For this review, take the finished solid that the model builds, in its own axes (mm). A direction names the side the tool comes from. Give positions to 0.01 mm unless a question says otherwise; leave off trailing zeros. Loops run counter-clockwise (first coordinate to the right, second up) from the corner with the lowest first, then second, coordinate; pieces in that order, holes last. Notation, with made-up numbers: (1, 26) -> (29, 26) arc R19 ccw to (29, 31) -> close; hole circle Ø3 at (-0.75, 37). An arc over 180 degrees is marked (long way). One line per question, with ' | ' between items. Start each with the question number.
(1) Consider section A-A (y = 6.5). Write out the cut boundary in (x, z), and give its area (3 significant figures).
(2) Wall thickness on probe 1 along Z at (x, y) = (-5.5, 11.25); probe 2 along Z at (x, y) = (0.25, 10.5); probe 3 along X at (y, z) = (12.3, 6.25): over which ranges is each line inside the solid? List them lowest first.
(3) Tool access review of faces 1 (the flat face through (-1, 3, -6)), 2 (the cylindrical face through (0.13, 12.73, 5.26)), 3 (the cylindrical face through (-3.361, 4.473, 11.186)): name each direction out of +Z, -Z, +X, -X, +Y, -Y from which nothing blocks a thin tool from reaching the whole face with its end or side.
(4) Insertion check: P1, Ø1, axis at x = -5.5, y = 9.5, coming from the -Z side; P2, Ø3, axis at x = -3.5, y = 11, coming from the +Z side; P3, Ø0.6, axis at y = 13, z = 0.5, coming from the -X side. Each pin has a flat end and moves straight along its axis. Give the tip position at first contact, or say it passes through.
from build123d import *

# Parameters (mm, degrees)
SKETCH1_W                    = 8.5
SKETCH1_H                    = 14.5
CUT_EXTRUDE1_REACH           = 2.1
CUT_EXTRUDE2_REACH           = 2.1
CUT_EXTRUDE3_REACH           = 2.1
CUT_EXTRUDE4_REACH           = 2.1
F_2_0_2_DIAMETER_HOLE1_D     = 2
F_2_0_2_DIAMETER_HOLE1_DEPTH = 3
F_2_0_2_DIAMETER_HOLE2_D     = 2
F_2_0_2_DIAMETER_HOLE2_DEPTH = 3.5
F_2_0_2_DIAMETER_HOLE3_D     = 2
F_2_0_2_DIAMETER_HOLE3_DEPTH = 3
F_2_0_2_DIAMETER_HOLE4_D     = 2
F_2_0_2_DIAMETER_HOLE4_DEPTH = 3.5


with BuildPart() as part:
    # Sketch1 → Revolve1 (revolve)
    with BuildSketch(Plane(origin=(0, 0, 0), x_dir=(-1, 0, 0), z_dir=(0, 0, -1))):
        with Locations((-4.25, 7.25)):
            Rectangle(SKETCH1_W, SKETCH1_H)
    revolve(axis=Axis((0, 0, 0), (0, 1, 0)))

    # Sketch2 → Cut-Extrude1 (cut, up to next)
    with BuildSketch(Plane(origin=(-8.4, 0, 0), x_dir=(0, 0, -1), z_dir=(1, 0, 0)), mode=Mode.PRIVATE) as cut_extrude1_sk1:
        Polygon((0.9, 13.234042555), (0.9, 13.297872335), (0.649999993, 13.297872335), (0.649999993, 13.553191453), (0.587500007, 13.553191453), (0.587500007, 13.297872335), (0.3375, 13.297872335), (0.3375, 13.234042555), (0.587500007, 13.234042555), (0.587500007, 12.978723392), (0.649999993, 12.978723392), (0.649999993, 13.234042555), align=None)
    cut_extrude1_tool1 = extrude(cut_extrude1_sk1.sketch, amount=-CUT_EXTRUDE1_REACH, mode=Mode.PRIVATE) & part.part
    add(cut_extrude1_tool1.solids().sort_by_distance((-8.4, 13.265957, -0.61875))[0], mode=Mode.SUBTRACT)

    # Sketch3 → Cut-Extrude2 (cut, up to next)
    with BuildSketch(Plane.XY.offset(-8.4), mode=Mode.PRIVATE) as cut_extrude2_sk1:
        Polygon((1, 13.234042555), (1, 13.297872335), (0.749999993, 13.297872335), (0.749999993, 13.553191453), (0.687500007, 13.553191453), (0.687500007, 13.297872335), (0.4375, 13.297872335), (0.4375, 13.234042555), (0.687500007, 13.234042555), (0.687500007, 12.978723392), (0.749999993, 12.978723392), (0.749999993, 13.234042555), align=None)
    cut_extrude2_tool1 = extrude(cut_extrude2_sk1.sketch, amount=-CUT_EXTRUDE2_REACH, mode=Mode.PRIVATE) & part.part
    add(cut_extrude2_tool1.solids().sort_by_distance((0.71875, 13.265957, -8.4))[0], mode=Mode.SUBTRACT)

    # Sketch4 → Cut-Extrude3 (cut, up to next)
    with BuildSketch(Plane.XY.offset(-8.4), mode=Mode.PRIVATE) as cut_extrude3_sk1:
        Polygon((-0.875, 12.5), (-0.43749997, 13.106382996), (-3e-08, 12.5), (0.18749997, 12.5), (-0.34374997, 13.265957445), (0.18749997, 14), (-3e-08, 14), (-0.43749997, 13.393617004), (-0.875, 14), (-1.0625, 14), (-0.53125006, 13.265957445), (-1.0625, 12.5), align=None)
    cut_extrude3_tool1 = extrude(cut_extrude3_sk1.sketch, amount=-CUT_EXTRUDE3_REACH, mode=Mode.PRIVATE) & part.part
    add(cut_extrude3_tool1.solids().sort_by_distance((-0.4375, 13.242259, -8.4))[0], mode=Mode.SUBTRACT)

    # Sketch5 → Cut-Extrude4 (cut, up to next)
    with BuildSketch(Plane(origin=(-8.4, 0, 0), x_dir=(0, 0, -1), z_dir=(1, 0, 0)), mode=Mode.PRIVATE) as cut_extrude4_sk1:
        Polygon((-1.10000006, 14), (-0.6, 13.265957445), (-0.6, 12.5), (-0.4125, 12.5), (-0.4125, 13.265957445), (0.08749997, 14), (-0.10000003, 14), (-0.50625, 13.393617004), (-0.91250006, 14), align=None)
    cut_extrude4_tool1 = extrude(cut_extrude4_sk1.sketch, amount=-CUT_EXTRUDE4_REACH, mode=Mode.PRIVATE) & part.part
    add(cut_extrude4_tool1.solids().sort_by_distance((-8.4, 13.37564, 0.50625))[0], mode=Mode.SUBTRACT)

    # Sketch6 → Revolve2 (revolve)
    with BuildSketch(Plane(origin=(0, 2.49, 0), x_dir=(1, 0, 0), z_dir=(0, 1, 0))):
        Polygon((-6.537367948, -13.647813756), (-4.635254916, -14.265847744), (-2.552899345, -7.857016287), (-4.455012378, -7.238982298), align=None)
    revolve(axis=Axis((-4.635254916, 2.49, 14.265847744), (0.309016994, 0, -0.951056516)))

    # Ø2.0 (2) Diameter Hole1
    with Locations(Plane(origin=(0, 0, 0), x_dir=(-1, 0, 0), z_dir=(0, -1, 0))):
        with Locations((1.08530111, 6.155048456), (-5.87307888, -2.137625896)):
            Hole(F_2_0_2_DIAMETER_HOLE1_D / 2, depth=F_2_0_2_DIAMETER_HOLE1_DEPTH)

    # Ø2.0 (2) Diameter Hole2
    with Locations(Plane(origin=(0, 0, 0), x_dir=(-1, 0, 0), z_dir=(0, -1, 0))):
        with Locations((6.226216863, -0.544723392), (-3.584852727, -5.119700277), (-2.641364136, 5.664423669)):
            Hole(F_2_0_2_DIAMETER_HOLE2_D / 2, depth=F_2_0_2_DIAMETER_HOLE2_DEPTH)

    # Ø2.0 (2) Diameter Hole3
    with Locations(Plane(origin=(0, 14.5, 0), x_dir=(1, 0, 0), z_dir=(0, 1, 0))):
        with Locations((0, 6.25), (-5.412658774, -3.125)):
            Hole(F_2_0_2_DIAMETER_HOLE3_D / 2, depth=F_2_0_2_DIAMETER_HOLE3_DEPTH)

    # Ø2.0 (2) Diameter Hole4
    with Locations(Plane(origin=(0, 14.5, 0), x_dir=(1, 0, 0), z_dir=(0, 1, 0))):
        with Locations((0, -6.25), (5.412658774, 3.125), (-5.412658774, 3.125)):
            Hole(F_2_0_2_DIAMETER_HOLE4_D / 2, depth=F_2_0_2_DIAMETER_HOLE4_DEPTH)


solid = part.part
A:
1) outline: circle Ø17 at (0, 0) | area: 227 mm^2
2) probe 1: z = -6.48 to -4.12, -2.13 to 6.48 | probe 2: z = -8.5 to 8.5 | probe 3: x = -5.76 to -1, 1 to 5.76
3) face 1: -Y | face 2: +Y | face 3: none
4) P1: stops at z = -6.87 | P2: stops at z = 8.26 | P3: stops at x = -8.5
